Read the model definition and answer for the solid it produces. Units are mm, in the model's axes. A direction names the side the tool comes from. Give positions to 0.01 mm unless a question says otherwise; leave off trailing zeros. Write each loop counter-clockwise with the first axis right and the second up, starting at its lowest first coordinate (ties: lowest second). Pieces come first, ordered by that corner, then holes. Notation, with made-up numbers: M 11.25,53.25 L 46.25,53.25 A23 cw 46.25,90.25 Z; hole C 15.5,3 d11. An arc over 180 degrees is marked long. Put each result on its own line as item: value.
from build123d import *

# Parameters (mm, degrees)
SKETCH1_R           = 4.762499999999989
SKETCH1_R_2         = 4.762500000000005
BOSS_EXTRUDE1_DEPTH = 9.525
CHAMFER1_SIZE       = 88.89999999999999
CHAMFER1_SIZE2      = 6.20588556630559
CHAMFER2_SIZE       = 88.89999999999999
CHAMFER2_SIZE2      = 6.300746042301969
FILLET1_R           = 8.528649
CUT_EXTRUDE2_DEPTH  = 117.6635246642072
FILLET4_R           = 3.175
CUT_EXTRUDE3_REACH  = 119.909
FILLET5_R           = 12.7
FILLET6_R           = 12.7
SKETCH15_R          = 4.7624999999999975
CUT_EXTRUDE7_DEPTH  = 117.82072113018388
FILLET9_R           = 12.7
CUT_EXTRUDE8_REACH  = 121.538
FILLET10_R          = 12.7


with BuildPart() as part:
    # Sketch1 → Boss-Extrude1 (new body)
    # profile 1 of 3: a face of its own
    with BuildSketch(Plane.XY):
        Polygon((-28.50000000000001, 23.36447913627793), (-28.500000000000007, 17.01447913627793), (-1.421e-14, 17.01447913627793), (-1.388e-14, 36.06447913627791), (-25.877441230163292, 36.06447913627793), align=None)
        with Locations(Location((-12.700000000000017, 26.539479136277926, 0), (0, 0, 180))):
            Circle(SKETCH1_R, mode=Mode.SUBTRACT)
    # profile 2 of 3: a face of its own
    with BuildSketch(Plane.XY):
        Polygon((1.421e-14, -11.046434023496033), (-28.499999999999996, -11.046434023496033), (-28.499999999999996, -17.396434023496035), (-25.877441230163278, -30.09643402349603), (1.421e-14, -30.09643402349603), align=None)
        with Locations(Location((-12.699999999999989, -20.571434023496032, 0), (0, 0, 180))):
            Circle(SKETCH1_R_2, mode=Mode.SUBTRACT)
    # profile 3 of 3: a face of its own
    with BuildSketch(Plane.XY):
        Polygon((-28.500000000000007, 17.01447913627793), (-28.5, -11.046434023496033), (1.421e-14, -11.046434023496033), (-5.89e-15, 17.014479136277927), align=None)
    extrude(amount=BOSS_EXTRUDE1_DEPTH)

    # Sweep1: sweep along a path in Sketch4
    with BuildLine(Plane(origin=(0, -11.046434023496033, 0), x_dir=(1, 0, 0), z_dir=(0, 1, 0))) as sweep1_path:
        Line((-14.249999999999991, -9.525), (-5.144041152540681, -93.4757286489478))
        Line((-5.144041152540681, -93.4757286489478), (-3.7745316583277084, -106.10167193035296))
    # Sketch3 → Sweep1 (sweep)
    with BuildSketch(Plane.XY.offset(9.525)):
        Polygon((-28.499999999999996, -11.046434023496033), (1.388e-14, -11.046434023496033), (-1.388e-14, 17.01447913627793), (-28.50000000000001, 17.01447913627793), align=None)
    sweep(path=sweep1_path.line)

    # Chamfer1
    chamfer1_edges = [part.edges().sort_by_distance(p)[0] for p in [
        (10.475468341672286, 2.9840225563909506, 106.10167193035296),
    ]]
    chamfer1_side = [part.faces().sort_by_distance(p)[0] for p in [
        (5.237734170836156, 2.9840225563909497, 57.813335965176485),
    ]]
    chamfer(chamfer1_edges, length=CHAMFER1_SIZE, length2=CHAMFER1_SIZE2, reference=chamfer1_side[0])

    # Chamfer2
    chamfer2_edges = [part.edges().sort_by_distance(p)[0] for p in [
        (-18.02453165832772, 2.984022556390949, 106.10167193035296),
    ]]
    chamfer2_side = [part.faces().sort_by_distance(p)[0] for p in [
        (-23.26226582916385, 2.9840225563909497, 57.813335965176506),
    ]]
    chamfer(chamfer2_edges, length=CHAMFER2_SIZE, length2=CHAMFER2_SIZE2, reference=chamfer2_side[0])

    # Fillet1
    fillet1_edges = [part.edges().sort_by_distance(p)[0] for p in [
        (4.269582775366721, 2.984022556390949, 106.10167193035296),
        (-11.72378561602573, 2.984022556390949, 106.10167193035296),
    ]]
    fillet(fillet1_edges, radius=FILLET1_R)

    # Sketch6 → Cut-Extrude2 (cut, through all)
    with BuildSketch(Plane.ZY.offset(28.500000000000004)):
        Polygon((81.13920097504592, 8.003565976503973), (106.10167193035296, 12.697715932081872), (106.10167193035296, -6.352284067918128), (81.13920097504591, -11.046434023496026), (117.96042684070639, -22.85606140259037), (128.32769329374543, 30.37810454166645), (17.720068960516624, 36.90132837728653), (9.525, 17.01447913627794), align=None)
    extrude(amount=-CUT_EXTRUDE2_DEPTH, mode=Mode.SUBTRACT)

    # Fillet4
    fillet4_edges = [part.edges().sort_by_distance(p)[0] for p in [
        (-14.249999999999995, -11.046434023496033, 9.525),
        (-14.25000000000001, 17.01447913627793, 9.525),
    ]]
    fillet(fillet4_edges, radius=FILLET4_R)

    # Cut-Extrude3: up to this plane
    cut_extrude3_end = Plane(origin=(-1.02e-15, 5.153508696821327, 0.3242221424168255), z_dir=(0, -0.9980268393792456, -0.06278875598921893))
    # Sketch8 → Cut-Extrude3 (cut, up to the surface)
    with BuildSketch(Plane(origin=(-6.1e-15, 17.929113719354145, 2.255944834364728), x_dir=(1, 3.4e-16, 4e-17), z_dir=(0, 0.9921767086467868, 0.12484141467810073)), mode=Mode.PRIVATE) as cut_extrude3_sk1:
        with BuildLine():
            ThreePointArc((-6.960254723021977, -13.301909437066078), (-3.6571329134227537, -14.633550570696002), (-2.2011808134518622, -17.88379445084032))
            Line((-2.2011808134518622, -17.88379445084032), (-0.1706376662483526, -71.38713388044914))
            ThreePointArc((-0.1706376662483526, -71.38713388044914), (-1.4988527094483572, -74.87087067627415), (-4.929711575818469, -76.33024886667496))
            Line((-4.929711575818469, -76.33024886667496), (-9.56390547472291, -76.33024886667496))
            ThreePointArc((-9.56390547472291, -76.33024886667496), (-12.621598981127008, -75.21903859372955), (-14.252419863558515, -72.40395403030512))
            Line((-14.252419863558515, -72.40395403030512), (-23.79483884579154, -18.9006146006963))
            ThreePointArc((-23.79483884579154, -18.9006146006963), (-22.75761418401056, -15.006715930662008), (-19.10632445695593, -13.301909437066078))
            Line((-19.10632445695593, -13.301909437066078), (-6.960254723021977, -13.301909437066078))
        make_face()
    cut_extrude3_tool1 = split(extrude(cut_extrude3_sk1.sketch, amount=-CUT_EXTRUDE3_REACH, mode=Mode.PRIVATE), bisect_by=cut_extrude3_end, keep=Keep.BOTH, mode=Mode.PRIVATE)
    add(cut_extrude3_tool1.solids().sort_by_distance((-10.437775, 12.651733, 44.197908))[0], mode=Mode.SUBTRACT)

    # Fillet5
    fillet5_edges = [part.edges().sort_by_distance(p)[0] for p in [
        (-28.50000000000001, 23.36447913627793, 4.7625),
    ]]
    fillet(fillet5_edges, radius=FILLET5_R)

    # Fillet6
    fillet6_edges = [part.edges().sort_by_distance(p)[0] for p in [
        (-1.404e-14, 36.06447913627791, 4.7625),
        (-25.877441230163292, 36.06447913627793, 4.7625),
    ]]
    fillet(fillet6_edges, radius=FILLET6_R)

    # Sketch15 → Cut-Extrude7 (cut, through all)
    with BuildSketch(Plane(origin=(2.39e-15, -7.006748203781874, 1.317607012078891), x_dir=(1, 3.3e-16, -6e-17), z_dir=(0, 0.9827744470593327, -0.18480905336920886))):
        with Locations(Location((-5.144041152540709, -95.00998731918351, 0), (0, 0, 270))):
            Circle(SKETCH15_R)
    extrude(amount=-CUT_EXTRUDE7_DEPTH, mode=Mode.SUBTRACT)

    # Fillet9
    fillet9_edges = [part.edges().sort_by_distance(p)[0] for p in [
        (1.404e-14, -30.09643402349603, 4.7625),
        (-25.877441230163278, -30.09643402349603, 4.7625),
        (-28.499999999999996, -17.396434023496035, 4.7625),
    ]]
    fillet(fillet9_edges, radius=FILLET9_R)

    # Cut-Extrude8: up to this plane
    cut_extrude8_end = Plane(origin=(-3.9e-16, 1.9847734817922233, 0.12486784215105542), z_dir=(0, -0.9980268393792456, -0.06278875598921893))
    # Sketch16 → Cut-Extrude8 (cut, up to the surface)
    with BuildSketch(Plane.XZ.offset(11.046434023496033), mode=Mode.PRIVATE) as cut_extrude8_sk1:
        with BuildLine():
            Line((-19.021943533629052, 15.875), (-6.942808285990063, 15.874999999999996))
            ThreePointArc((-6.942808285990063, 15.874999999999996), (-3.6401991085921965, 17.206147661436145), (-2.183788559280739, 20.455462941157986))
            Line((-2.183788559280739, 20.455462941157986), (-0.17315756899978269, 73.01966391620381))
            ThreePointArc((-0.17315756899978269, 73.01966391620381), (-1.5008249571452126, 76.50431015244372), (-4.932177295709103, 77.9642009750459))
            Line((-4.932177295709103, 77.9642009750459), (-9.573100570431755, 77.9642009750459))
            ThreePointArc((-9.573100570431755, 77.9642009750459), (-12.628305718550124, 76.85507308214247), (-14.260471182334522, 74.04429399464112))
            Line((-14.260471182334522, 74.04429399464112), (-23.709314145531817, 21.480093019595273))
            ThreePointArc((-23.709314145531817, 21.480093019595273), (-22.67531564072565, 17.582294851881656), (-19.021943533629052, 15.875))
        make_face()
    cut_extrude8_tool1 = split(extrude(cut_extrude8_sk1.sketch, amount=-CUT_EXTRUDE8_REACH, mode=Mode.PRIVATE), bisect_by=cut_extrude8_end, keep=Keep.BOTH, mode=Mode.PRIVATE)
    add(cut_extrude8_tool1.solids().sort_by_distance((-10.411854, -11.046434, 44.429711))[0], mode=Mode.SUBTRACT)

    # Fillet10
    fillet10_edges = [part.edges().sort_by_distance(p)[0] for p in [
        (-6.448124287799661, -11.046434023496028, 81.13920097504591),
    ]]
    fillet(fillet10_edges, radius=FILLET10_R)


solid = part.part
(1) Given pin 1 Ø9.5 at (x, y) = (-12, -8) entering from +Z; pin 2 Ø9.5 at (x, z) = (-11, 57) entering from -Y; pin 3 Ø18 at (x, y) = (-13.5, 25) entering from +Z, each flat-ended and moving along its own axis, determine where each tip first touches the part or whether it passes through.
Result:
pin 1: stops at z = 105.59
pin 2: stops at y = -1.89
pin 3: stops at z = 15.45
(2) Section C-C on z = 67 is taken. Determine the outline of the cut face in (x, y), and give its area (3 significant figures).
Result:
outline: M -18.75,-11.05 L -15.53,-11.05 L -15.53,-2.22 L -0.4,-2.22 L -0.4,-11.05 L 2.77,-11.05 L 2.77,9.78 L -0.4,9.78 L -0.36,0.96 L -15.33,0.96 L -15.53,9.78 L -18.75,9.78 Z
area: 182 mm²
(3) Section B-B on x = -22.5 is taken. Determine the outline of the cut face in (y, z) (3 decimals).
Result:
outline: M -28.014,0 L 33.982,0 L 33.982,9.525 L 19.815,9.525 A3.175 cw 16.665,12.304 L 16.091,16.864 L 4.207,15.369 L 3.487,26.806 L 14.663,28.212 L 12.406,46.153 L -11.046,46.153 L -11.046,28.208 L 0.218,28.208 L 0.899,17.384 L -11.046,17.384 L -11.046,12.7 A3.175 cw -14.221,9.525 L -28.014,9.525 Z
(4) Which of the six approach directions +Z, -Z, +X, -X, +Y, -Y give full straight-line access (tool end or side, diameter ignored) to faces 1 (the face through (-14, -30.096, 5)), 2 (the face through (-7.21, 4.42, 77.49)), 3 (the face through (-22.712, -5.111, 17.627)), 4 (the face through (0, 3, 5))?
Result:
face 1: +Z, -Z, +X, -X, -Y
face 2: +Y
face 3: -Y
face 4: -Z, +X, +Y, -Y
(5) Section A-A on z = 36.5 is taken. Determine the outline of the cut face in (x, y).
Result:
outline: M -24.24,-11.05 L -21.01,-11.05 L -21.01,-0.3 L -1.57,-0.3 L -1.57,-11.05 L 1.61,-11.05 L 1.61,13.62 L -1.57,13.62 L -1.52,2.88 L -20.77,2.88 L -21.01,13.62 L -24.24,13.62 Z
(6) For a pull along X with two mould halves and no side action, classify faces 5 (the face through (-3.819, 32.443, 4.829)), 6 (the face through (-0.844, 12.354, 46.561)), 7 (the face through (-1.193, -6.558, 46.37)) as +X half, -X half, draft (parallel to the pull), parting line (faces both ways), or undercut.
Result:
face 5: +X half
face 6: draft
face 7: undercut
(7) Straight lines are drawn through the part: line 1 along Z through (x, y) = (-5, 7); line 2 along Y through (x, z) = (-12, 7); line 3 along X through (y, z) = (7.5, 8.5). For each, find the intervals that lie inside material, in ascending order. Write a range as from..to.
Result:
line 1: z = 0..14.71, 77.81..90.52, 100.2..106.09
line 2: y = -30.08..-25.28, -15.86..21.83, 31.25..36.05
line 3: x = -28.5..0
